Can you work these out from the model? Positions are in its coordinate system, mm. A direction names the side the tool comes from. Round coordinates to 2 decimals unless told otherwise and drop trailing zeros. Order: outer loops, then holes, each group sorted by start corner. A loop starts at its lowest first (then second) coordinate and runs counter-clockwise, first axis right, second up.
from build123d import *

# Parameters (mm, degrees)
SKETCH1_R           = 39.6875
BOSS_EXTRUDE1_DEPTH = 25.4
SHELL1_T            = -2.54
CUT_EXTRUDE1_DEPTH  = 62.60645512
SKETCH4_R           = 12.124567064
CUT_EXTRUDE2_DEPTH  = 0.254
FILLET1_R           = 3.175
SKETCH5_R           = 2.38125
CUT_EXTRUDE3_DEPTH  = 62.606455185
FILLET2_R           = 3.175


with BuildPart() as part:
    # Sketch1 → Boss-Extrude1 (new body)
    with BuildSketch(Plane(origin=(0, 0, 0), x_dir=(1, 0, 0), z_dir=(0, 1, 0))):
        with Locations(Location((0, 0, 0), (0, 0, 270))):
            Circle(SKETCH1_R)
    extrude(amount=BOSS_EXTRUDE1_DEPTH)

    # Shell1
    shell1_openings = [part.faces().sort_by_distance(p)[0] for p in [
        (0, 25.4, 0),
    ]]
    offset(amount=SHELL1_T, openings=shell1_openings, kind=Kind.INTERSECTION)

    # Sketch2 → Cut-Extrude1 (cut, through all)
    with BuildSketch(Plane(origin=(0, 25.4, 0), x_dir=(1, 0, 0), z_dir=(0, 1, 0))):
        Polygon((-5.55625, 10.776512071), (5.55625, 10.776512071), (12.124567064, 0), (5.55625, -10.776512071), (-5.55625, -10.776512071), (-12.124567064, 0), align=None)
    extrude(amount=-CUT_EXTRUDE1_DEPTH, mode=Mode.SUBTRACT)

    # Sketch4 → Cut-Extrude2 (cut)
    with BuildSketch(Plane(origin=(0, 2.54, 0), x_dir=(1, 0, 0), z_dir=(0, 1, 0))):
        with Locations(Location((0, 0, 0), (0, 0, 270))):
            Circle(SKETCH4_R)
    extrude(amount=-CUT_EXTRUDE2_DEPTH, mode=Mode.SUBTRACT)

    # Fillet1
    fillet1_edges = [part.edges().sort_by_distance(p)[0] for p in [
        (0, 0, -39.6875),
    ]]
    fillet(fillet1_edges, radius=FILLET1_R)

    # Sketch5 → Cut-Extrude3 (cut, through all)
    with BuildSketch(Plane.XZ):
        with Locations(Location((19.866785326, 20.619012071, 0), (0, 0, 270))):
            Circle(SKETCH5_R)
        with Locations(Location((-18.413118107, 20.619012071, 0), (0, 0, 270))):
            Circle(SKETCH5_R)
        with Locations(Location((-18.413118107, -20.619012071, 0), (0, 0, 270))):
            Circle(SKETCH5_R)
        with Locations(Location((19.866785326, -17.126512071, 0), (0, 0, 270))):
            Circle(SKETCH5_R)
    extrude(amount=-CUT_EXTRUDE3_DEPTH, mode=Mode.SUBTRACT)

    # Fillet2
    fillet2_edges = [part.edges().sort_by_distance(p)[0] for p in [
        (0, 2.54, -37.1475),
    ]]
    fillet(fillet2_edges, radius=FILLET2_R)


solid = part.part
(1) On a 3-axis mill with a long thin cutter (end or side, diameter ignored), from which of +Z, -Z, +X, -X, +Y, -Y can I reach the whole of each face in a straight line? I mean faces 1 (the face through (-8.89, 1.16, -5.31)), 2 (the face through (10, 2.286, -6)), 3 (the face through (-8, 0, 8)). Say none if no direction works.
(2) I want a section at B-B, the plane y = 16. List the corners of the cut face in (x, z) for me (1 decimal).
(3) I want a section at C-C, the plane y = 4.75. List the corners of the cut face in (x, z) for me (1 decimal).
(4) Please list where these lines run through material, in increasing order: probe 1 along Y at (x, z) = (24.5, -18); probe 2 along X at (y, z) = (12.5, -3.5); probe 3 along Z at (x, y) = (27.5, 12).
(5) I'm going to push flat-ended pins straight in: pin 1 Ø8 at (y, z) = (3.5, -25.5) entering from -X; pin 2 Ø4 at (x, z) = (-18.41, 20.62) entering from -Y; pin 3 Ø3 at (x, y) = (3.5, 2.5) entering from -Z; pin 4 Ø5 at (x, z) = (-15, 1) entering from +Y. Where does each tip first touch, or does it pass through?
Ans:
1. face 1: +Y, -Y
1. face 2: +Y
1. face 3: +Z, -Z, +X, -X, -Y
2. outline: circle Ø79.4 at (0, 0); hole circle Ø74.3 at (0, 0)
3. outline: circle Ø79.4 at (0, 0); hole circle Ø74 at (0, 0)
4. probe 1: y = 0 to 2.54
4. probe 2: x = -39.53 to -36.98, 36.98 to 39.53
4. probe 3: z = -28.62 to -24.97, 24.97 to 28.62
5. pin 1: stops at x = -33.36
5. pin 2: passes through
5. pin 3: stops at z = -39.63
5. pin 4: stops at y = 2.54
